```python
from build123d import *

# Parameters (mm, degrees)
SKETCH_1_R      = 80
SKETCH_1_R_2    = 1.52
SKETCH_1_R_3    = 2.025
SKETCH_1_R_4    = 1.6
SKETCH_1_W      = 15
SKETCH_1_H      = 25
EXTRUDE_1_DEPTH = 3
SKETCH_1103_W   = 7
SKETCH_1103_H   = 3.2
SKETCH_1103_W_2 = 3.2
SKETCH_1103_H_2 = 7
BB_DEPTH        = 3
FILLET_1_R      = 3


with BuildPart() as part:
    # 草图1 → 凸台-拉伸1 (new body)
    with BuildSketch(Plane.XY):
        Circle(SKETCH_1_R)
        with Locations((-47, 47)):
            Circle(SKETCH_1_R_2, mode=Mode.SUBTRACT)
        with Locations((47, 47)):
            Circle(SKETCH_1_R_2, mode=Mode.SUBTRACT)
        with Locations((47, -47)):
            Circle(SKETCH_1_R_2, mode=Mode.SUBTRACT)
        with Locations((-47, -47)):
            Circle(SKETCH_1_R_2, mode=Mode.SUBTRACT)
        with Locations((19, 60)):
            Circle(SKETCH_1_R_3, mode=Mode.SUBTRACT)
        with Locations((15, 72)):
            Circle(SKETCH_1_R_3, mode=Mode.SUBTRACT)
        with Locations((15, 48)):
            Circle(SKETCH_1_R_3, mode=Mode.SUBTRACT)
        with Locations((-15, 48)):
            Circle(SKETCH_1_R_3, mode=Mode.SUBTRACT)
        with Locations((-19, 60)):
            Circle(SKETCH_1_R_3, mode=Mode.SUBTRACT)
        with Locations((-15, 72)):
            Circle(SKETCH_1_R_3, mode=Mode.SUBTRACT)
        with Locations((15, -48)):
            Circle(SKETCH_1_R_3, mode=Mode.SUBTRACT)
        with Locations((15, -72)):
            Circle(SKETCH_1_R_3, mode=Mode.SUBTRACT)
        with Locations((19, -60)):
            Circle(SKETCH_1_R_3, mode=Mode.SUBTRACT)
        with Locations((-15, -48)):
            Circle(SKETCH_1_R_3, mode=Mode.SUBTRACT)
        with Locations((-19, -60)):
            Circle(SKETCH_1_R_3, mode=Mode.SUBTRACT)
        with Locations((-15, -72)):
            Circle(SKETCH_1_R_3, mode=Mode.SUBTRACT)
        with Locations((-35, 62.5)):
            Circle(SKETCH_1_R_4, mode=Mode.SUBTRACT)
        with Locations((-35, -62.5)):
            Circle(SKETCH_1_R_4, mode=Mode.SUBTRACT)
        with Locations((-31.5, 8.5)):
            Circle(SKETCH_1_R_4, mode=Mode.SUBTRACT)
        with Locations((-31.5, -8.5)):
            Circle(SKETCH_1_R_4, mode=Mode.SUBTRACT)
        with Locations((31.5, -8.5)):
            Circle(SKETCH_1_R_4, mode=Mode.SUBTRACT)
        with Locations((31.5, 8.5)):
            Circle(SKETCH_1_R_4, mode=Mode.SUBTRACT)
        with Locations((35, 62.5)):
            Circle(SKETCH_1_R_4, mode=Mode.SUBTRACT)
        with Locations((35, -62.5)):
            Circle(SKETCH_1_R_4, mode=Mode.SUBTRACT)
        with Locations((0, -32.5)):
            Rectangle(SKETCH_1_W, SKETCH_1_H, mode=Mode.SUBTRACT)
    extrude(amount=EXTRUDE_1_DEPTH)

    # Sketch 1103 → 电池+BB响扎带孔位 (cut)
    with BuildSketch(Plane.XY):
        with Locations((20, -20)):
            Rectangle(SKETCH_1103_W, SKETCH_1103_H)
        with Locations((20, 20)):
            Rectangle(SKETCH_1103_W, SKETCH_1103_H)
        with Locations((55, 0)):
            Rectangle(SKETCH_1103_W_2, SKETCH_1103_H_2)
        with Locations((-20, 20)):
            Rectangle(SKETCH_1103_W, SKETCH_1103_H)
        with Locations((-55, 0)):
            Rectangle(SKETCH_1103_W_2, SKETCH_1103_H_2)
        with Locations((-20, -20)):
            Rectangle(SKETCH_1103_W, SKETCH_1103_H)
    extrude(amount=BB_DEPTH, mode=Mode.SUBTRACT)

    # 圆角1
    fillet_1_edges = [part.edges().sort_by_distance(p)[0] for p in [
        (-7.5, -20, 1.5),
        (-7.5, -45, 1.5),
        (7.5, -45, 1.5),
        (7.5, -20, 1.5),
    ]]
    fillet(fillet_1_edges, radius=FILLET_1_R)


solid = part.part
```
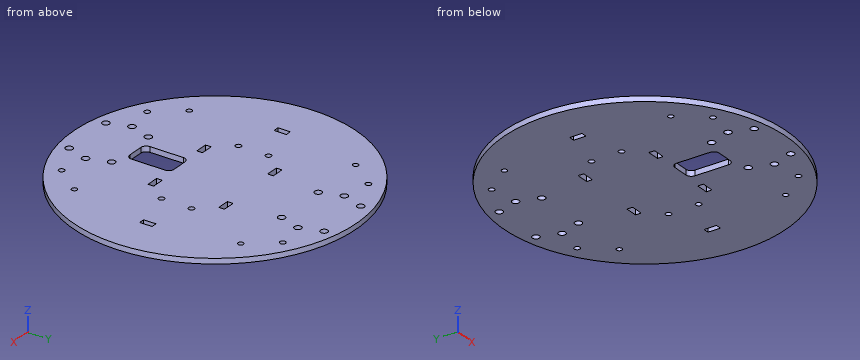
For this review, take the finished solid that the model builds, in its own axes (mm). Coordinates: 2 decimals unless noted, no trailing zeros. Order: outer loops, then holes, each group sorted by start corner. A loop starts at its lowest first (then second) coordinate and runs counter-clockwise, first axis right, second up. Notation, with made-up numbers: (82, 21.25) -> (132, 21.25) arc R32 ccw to (132, 57.25) -> close; hole circle Ø9 at (36.25, 68.5). An arc over 180 degrees is marked (long way). Use CSV: the item, a comma, the result in double quotes. Start each with the question number.
Item 1: We need section B-B, the plane y = 72. Give the boundary of the cut face in (x, z) (3 decimals).
Item 2: Wall thickness on probe 1 along Y at (x, z) = (-15, 0.85) (3 decimals); probe 2 along Y at (x, z) = (35, 1.4); probe 3 along X at (y, z) = (21, 2.4): over which ranges is each line inside the solid? List them lowest first.
Item 3: We need section C-C, the plane x = -19. Give the boundary of the cut face in (y, z) (3 decimals), then the cut area to 3 significant figures.
Item 4: We need section A-A, the plane x = 2. Give the boundary of the cut face in (y, z) (3 decimals), then the cut area to 3 significant figures.
Item 5: Insertion check: pin 1 (1.5 mm diameter, centred on x = 54.5, z = 1, fed in from -Y); pin 2 (1.5 mm diameter, centred on x = 19.5, z = 2, fed in from +Y); pin 3 (1.5 mm diameter, centred on y = -21, z = 1, fed in from -X). Each pin has a flat end and moves straight along its axis. Give the tip position at first contact, or say it passes through.
Item 6: We need section D-D, the plane y = -26. Give the boundary of the cut face in (x, z).
Derived:
1,outline,"(-34.871, 0) -> (-17.025, 0) -> (-17.025, 3) -> (-34.871, 3) -> close; (-12.975, 0) -> (12.975, 0) -> (12.975, 3) -> (-12.975, 3) -> close; (17.025, 0) -> (34.871, 0) -> (34.871, 3) -> (17.025, 3) -> close"
2,probe 1,"y = -78.581 to -74.025, -69.975 to -50.025, -45.975 to 45.975, 50.025 to 69.975, 74.025 to 78.581"
2,probe 2,"y = -71.94 to -64.1, -60.9 to 60.9, 64.1 to 71.94"
2,probe 3,"x = -77.19 to -23.5, -16.5 to 16.5, 23.5 to 77.19"
3,outline,"(-77.711, 0) -> (-62.025, 0) -> (-62.025, 3) -> (-77.711, 3) -> close; (-57.975, 0) -> (-21.6, 0) -> (-21.6, 3) -> (-57.975, 3) -> close; (-18.4, 0) -> (18.4, 0) -> (18.4, 3) -> (-18.4, 3) -> close; (21.6, 0) -> (57.975, 0) -> (57.975, 3) -> (21.6, 3) -> close; (62.025, 0) -> (77.711, 0) -> (77.711, 3) -> (62.025, 3) -> close"
3,area,"423 mm^2"
4,outline,"(-79.975, 0) -> (-45, 0) -> (-45, 3) -> (-79.975, 3) -> close; (-20, 0) -> (79.975, 0) -> (79.975, 3) -> (-20, 3) -> close"
4,area,"405 mm^2"
5,pin 1,"stops at y = -59.25"
5,pin 2,"stops at y = 77.77"
5,pin 3,"stops at x = -77.39"
6,outline,"(-75.66, 0) -> (-7.5, 0) -> (-7.5, 3) -> (-75.66, 3) -> close; (7.5, 0) -> (75.66, 0) -> (75.66, 3) -> (7.5, 3) -> close"
